Could you check a few things on this model? Use its own coordinates, in mm. Face numbers are marked on the shaded views. A direction names the side the tool comes from. Coordinates: 2 decimals unless noted, no trailing zeros. Order: outer loops, then holes, each group sorted by start corner. A loop starts at its lowest first (then second) coordinate and runs counter-clockwise, first axis right, second up. Notation, with made-up numbers: (8.25, 33.5) - (22.25, 33.5) arc R9 cw to (22.25, 45.5) - close; hole circle Ø10 at (-14, 29). An arc over 180 degrees is marked (long way). Answer as CSV lines item,"result". Start each with the question number.
1. I need wall thicknesses on probe 1 along Z at (x, y) = (-20, -2); probe 2 along Y at (x, z) = (0, 5); probe 3 along Y at (x, z) = (13.5, 0.5). Which ranges of each line are inside material? Lowest first, please.
2. For the marked faces 1 and 2, which set-ups out of +Z, -Z, +X, -X, +Y, -Y let a thin tool reach every point of the face, with its end or its side?
3. For pin 1 (1.5 mm diameter, centred on y = 4, z = 7.5, fed in from +X); pin 2 (2 mm diameter, centred on x = -2.5, z = 7, fed in from -Y); pin 3 (1 mm diameter, centred on y = -1.5, z = 4.5, fed in from +X), each with a flat end and sliding along its axis, tell me the tip position at first contact or that it passes through.
4. I want a section at A-A, the plane x = 0. List the corners of the cut face in (y, z) for me, and give its area (4 significant figures).
5. I want a section at B-B, the plane y = -5.5. List the corners of the cut face in (x, z) for me, and give its area (4 significant figures).
6. I want a section at C-C, the plane z = 9.5. List the corners of the cut face in (x, y) for me.
from build123d import *

# Parameters (mm, degrees)
SKETCH1_W           = 45
SKETCH1_H           = 45
BOSS_EXTRUDE1_DEPTH = 2.5
FILLET1_R           = 1
SKETCH2_R           = 4
BOSS_EXTRUDE2_DEPTH = 10
CHAMFER1_SIZE       = 1


with BuildPart() as part:
    # Sketch1 → Boss-Extrude1 (new body)
    with BuildSketch(Plane.XY):
        Rectangle(SKETCH1_W, SKETCH1_H)
    extrude(amount=BOSS_EXTRUDE1_DEPTH)

    # Fillet1
    fillet1_edges = [part.edges().sort_by_distance(p)[0] for p in [
        (-22.5, 22.5, 1.25),
        (22.5, 22.5, 1.25),
        (22.5, -22.5, 1.25),
        (-22.5, -22.5, 1.25),
    ]]
    fillet(fillet1_edges, radius=FILLET1_R)

    # Sketch2 → Boss-Extrude2 (add)
    with BuildSketch(Plane.XY.offset(2.5)):
        Circle(SKETCH2_R)
    extrude(amount=BOSS_EXTRUDE2_DEPTH)

    # Chamfer1
    chamfer1_edges = [part.edges().sort_by_distance(p)[0] for p in [
        (0, -22.5, 0),
        (-22.5, 0, 0),
        (0, 22.5, 0),
        (22.5, 0, 0),
        (22.207106781, 22.207106781, 0),
        (-22.207106781, 22.207106781, 0),
        (22.207106781, -22.207106781, 0),
        (-22.207106781, -22.207106781, 0),
    ]]
    chamfer(chamfer1_edges, length=CHAMFER1_SIZE)


solid = part.part
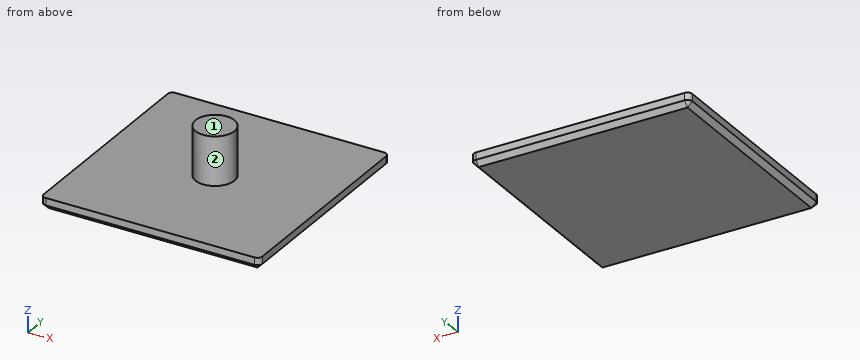
Solved:
1,probe 1,"z = 0 to 2.5"
1,probe 2,"y = -4 to 4"
1,probe 3,"y = -22 to 22"
2,face 1,"+Z, +X, -X, +Y, -Y"
2,face 2,"+Z"
3,pin 1,"stops at x = 2.33"
3,pin 2,"stops at y = -3.71"
3,pin 3,"stops at x = 3.87"
4,outline,"(-22.5, 1) - (-21.5, 0) - (21.5, 0) - (22.5, 1) - (22.5, 2.5) - (4, 2.5) - (4, 12.5) - (-4, 12.5) - (-4, 2.5) - (-22.5, 2.5) - close"
4,area,"191.5 mm2"
5,outline,"(-22.5, 1) - (-21.5, 0) - (21.5, 0) - (22.5, 1) - (22.5, 2.5) - (-22.5, 2.5) - close"
5,area,"111.5 mm2"
6,outline,"circle Ø8 at (0, 0)"
